Geometry check sheet. Reference: the model listing, model coordinates, mm. Face numbers are marked on the shaded views. A direction names the side the tool comes from. Give positions to 0.01 mm unless a question says otherwise; leave off trailing zeros. Order: outer loops, then holes, each group sorted by start corner. A loop starts at its lowest first (then second) coordinate and runs counter-clockwise, first axis right, second up.
from build123d import *

# Parameters (mm, degrees)
SKETCH1_R           = 11
BOSS_EXTRUDE1_DEPTH = 7
SKETCH3_R           = 18.5
CUT_EXTRUDE1_DEPTH  = 8
CUT_EXTRUDE2_DEPTH  = 2.9
CUT_EXTRUDE3_DEPTH  = 8
SKETCH7_R           = 1.5
CUT_EXTRUDE4_DEPTH  = 5.1
SKETCH10_R          = 2
CUT_EXTRUDE5_DEPTH  = 8


with BuildPart() as part:
    # Sketch1 → Boss-Extrude1 (new body)
    with BuildSketch(Plane.XY):
        with BuildLine():
            Line((42.143593539, 104.994845224), (-13.856406461, 8))
            ThreePointArc((-13.856406461, 8), (-13.856406461, -8), (0, -16))
            Line((0, -16), (112, -16))
            ThreePointArc((112, -16), (125.856406461, -8), (125.856406461, 8))
            Line((125.856406461, 8), (69.856406461, 104.994845224))
            ThreePointArc((69.856406461, 104.994845224), (56, 112.994845224), (42.143593539, 104.994845224))
        make_face()
        Circle(SKETCH1_R, mode=Mode.SUBTRACT)
        with Locations((112, 0)):
            Circle(SKETCH1_R, mode=Mode.SUBTRACT)
        with Locations((56, 96.994845224)):
            Circle(SKETCH1_R, mode=Mode.SUBTRACT)
    extrude(amount=BOSS_EXTRUDE1_DEPTH)

    # Sketch3 → Cut-Extrude1 (cut, through all)
    with BuildSketch(Plane.XY.offset(7)):
        with Locations((56, 65.944845224)):
            Circle(SKETCH3_R)
    extrude(amount=-CUT_EXTRUDE1_DEPTH, mode=Mode.SUBTRACT)

    # Sketch4 → Cut-Extrude2 (cut)
    with BuildSketch(Plane.XY.offset(7)):
        with BuildLine():
            Line((44.91, 82.494845224), (65.74, 82.494845224))
            Line((65.74, 82.494845224), (67.963130932, 88.602847259))
            Line((67.963130932, 88.602847259), (78.535172855, 87.67791344))
            Line((78.535172855, 87.67791344), (75.282447168, 42.324405576))
            Line((75.282447168, 42.324405576), (55.030844768, 27.665872217))
            Line((55.030844768, 27.665872217), (38.701277947, 54.952961607))
            Line((38.701277947, 54.952961607), (30.604248297, 78.605405685))
            ThreePointArc((30.604248297, 78.605405685), (32.46849594, 85.181842037), (39.280834875, 85.744845224))
            Line((39.280834875, 85.744845224), (44.91, 82.494845224))
        make_face()
    extrude(amount=-CUT_EXTRUDE2_DEPTH, mode=Mode.SUBTRACT)

    # Sketch5 → Cut-Extrude3 (cut, through all)
    with BuildSketch(Plane.XY.offset(7)):
        with BuildLine():
            Line((22.59151766, 41.129656408), (9.622063078, 18.665902125))
            ThreePointArc((9.622063078, 18.665902125), (19.321434948, 8.226916285), (20.124611797, -6))
            Line((20.124611797, -6), (49.031546624, -6))
            Line((49.031546624, -6), (49.031546624, 18.216961725))
            Line((49.031546624, 18.216961725), (35.260372543, 41.228916805))
            ThreePointArc((35.260372543, 41.228916805), (28.939452074, 39.455357607), (22.59151766, 41.129656408))
        make_face()
        with BuildLine():
            Line((59.031546624, 18.216961725), (59.031546624, -6))
            Line((59.031546624, -6), (91.875388203, -6))
            ThreePointArc((91.875388203, -6), (92.678565052, 8.226916285), (102.377936922, 18.665902125))
            Line((102.377936922, 18.665902125), (96.035225677, 29.651800259))
            ThreePointArc((96.035225677, 29.651800259), (87.175426517, 28.252595389), (79.659424477, 33.147851127))
            Line((79.659424477, 33.147851127), (59.031546624, 18.216961725))
        make_face()
    extrude(amount=-CUT_EXTRUDE3_DEPTH, mode=Mode.SUBTRACT)

    # Sketch7 → Cut-Extrude4 (cut, through all)
    with BuildSketch(Plane.XY.offset(4.1)):
        with Locations((68.100893251, 42.839462205)):
            Circle(SKETCH7_R)
        with Locations((36.41, 79.994845224)):
            Circle(SKETCH7_R)
    extrude(amount=-CUT_EXTRUDE4_DEPTH, mode=Mode.SUBTRACT)

    # Sketch10 → Cut-Extrude5 (cut, through all)
    with BuildSketch(Plane.XY.offset(7)):
        with Locations((24.388784068, 59.24261314)):
            Circle(SKETCH10_R)
        with Locations((16.888784068, 46.252232084)):
            Circle(SKETCH10_R)
        with Locations((87.611215932, 59.24261314)):
            Circle(SKETCH10_R)
        with Locations((95.111215932, 46.252232084)):
            Circle(SKETCH10_R)
    extrude(amount=-CUT_EXTRUDE5_DEPTH, mode=Mode.SUBTRACT)


solid = part.part
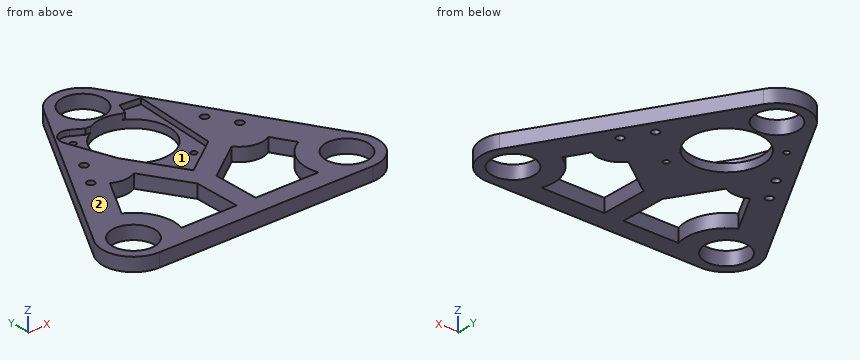
Item 1: Set-up check for the marked faces 1 and 2: record each of +Z, -Z, +X, -X, +Y, -Y from which the full face is reachable in a straight line by a thin tool's end or side.
Reported:
face 1: +Z
face 2: +Z, +X, -X, +Y, -Y
Item 2: Gauge pin test, flat ends, axial feed: pin 1 (2 mm diameter, centred on x = 58, z = 1.5, fed in from +Y); pin 2 (1.5 mm diameter, centred on y = 90.5, z = 3.5, fed in from -X); pin 3 (2 mm diameter, centred on x = 81, z = 5, fed in from +Y). Record the tip position at first contact, or that the pin passes through.
Reported:
pin 1: stops at y = 112.96
pin 2: stops at x = 33.34
pin 3: stops at y = 87.43
Item 3: Scan lines: L1, parallel to Y at x = 49, z = 2.5; L2, parallel to Y at x = 36.41, z = 2.75; L3, parallel to Y at x = 72, z = 5.5. Record each from-to range of solid material in increasing order.
Reported:
L1: y = -16 to -6, 18.27 to 48.82, 83.07 to 88.51, 105.48 to 111.38
L2: y = -16 to -6, 39.31 to 78.49, 81.49 to 95.06
L3: y = -16 to -6, 27.6 to 39.95, 88.25 to 101.28
Item 4: Sectioned sample at C-C (y = 35). Enter the section's corners in (x, z), and give its area (3 significant figures).
Reported:
outline: (1.73, 0) - (19.05, 0) - (19.05, 7) - (1.73, 7) - close; (38.99, 0) - (110.27, 0) - (110.27, 7) - (65.16, 7) - (65.16, 4.1) - (50.64, 4.1) - (50.64, 7) - (38.99, 7) - close
area: 578 mm2
Item 5: Sectioned sample at D-D (y = 15). Enter the section's corners in (x, z), and give its area (3 significant figures).
Reported:
outline: (-9.81, 0) - (14.7, 0) - (14.7, 7) - (-9.81, 7) - close; (49.03, 0) - (59.03, 0) - (59.03, 7) - (49.03, 7) - close; (97.3, 0) - (121.81, 0) - (121.81, 7) - (97.3, 7) - close
area: 413 mm2
Item 6: Sectioned sample at A-A (y = 0). Enter the section's corners in (x, z), and give its area (3 significant figures).
Reported:
outline: (-16, 0) - (-11, 0) - (-11, 7) - (-16, 7) - close; (11, 0) - (21, 0) - (21, 7) - (11, 7) - close; (49.03, 0) - (59.03, 0) - (59.03, 7) - (49.03, 7) - close; (91, 0) - (101, 0) - (101, 7) - (91, 7) - close; (123, 0) - (128, 0) - (128, 7) - (123, 7) - close
area: 280 mm2
Item 7: Sectioned sample at B-B (z = 2.5). Give the number of separate pieces and of enclosed holes in the cut face, and give its area (3 significant figures).
Reported:
separate pieces: 1
enclosed holes: 12
area: 6,810 mm2
